from build123d import *

# Parameters (mm, degrees)
SKETCH7_R           = 15.75
BOSS_EXTRUDE5_DEPTH = 2
SKETCH8_R           = 0.8
BOSS_EXTRUDE6_DEPTH = 5


with BuildPart() as part:
    # Sketch7 → Boss-Extrude5 (new body)
    with BuildSketch(Plane(origin=(0, 0, 0), x_dir=(1, 0, 0), z_dir=(0, 1, 0))):
        with Locations(Location((0, 0, 0), (0, 0, 270))):
            Circle(SKETCH7_R)
    extrude(amount=BOSS_EXTRUDE5_DEPTH)

    # Sketch8 → Boss-Extrude6 (add)
    with BuildSketch(Plane.XZ):
        with Locations(Location((0, 14, 0), (0, 0, 90))):
            Circle(SKETCH8_R)
        with Locations(Location((14, 0, 0), (0, 0, 90))):
            Circle(SKETCH8_R)
        with Locations(Location((0, -14, 0), (0, 0, 90))):
            Circle(SKETCH8_R)
        with Locations(Location((-14, 0, 0), (0, 0, 90))):
            Circle(SKETCH8_R)
    extrude(amount=BOSS_EXTRUDE6_DEPTH)


solid = part.part
The listing builds one solid part. Answer for the finished solid, in the listing's coordinates (mm). A direction names the side the tool comes from. Round coordinates to 2 decimals unless told otherwise and drop trailing zeros. Write each loop counter-clockwise with the first axis right and the second up, starting at its lowest first coordinate (ties: lowest second). Pieces come first, ordered by that corner, then holes. Notation, with made-up numbers: (38.5, 56.5) - (77.5, 56.5) arc R13 cw to (77.5, 69.5) - close; hole circle Ø2 at (49, 19.5). An arc over 180 degrees is marked (long way). Use a Markdown table: item, result. Add a question column.
1. For a pull along Z with two mould halves and no side action, classify faces 3 (the face through (-14, -5, 0)), 4 (the face through (-0.54, -2.46, -14.59)), 5 (the face through (13.207, -2.465, -0.104)) as +Z half, -Z half, draft (parallel to the pull), parting line (faces both ways), or undercut.
2. The part is cut by section B-B (z = 0). Write down the section's boundary in (x, y), and give its area (3 significant figures).
3. A tool of negligible diameter and unlimited length cuts with its end or side. For faces 1 (the face through (15.616, 0.986, -2.05)), 2 (the face through (-0.54, -2.46, 13.41)), from which of +Z, -Z, +X, -X, +Y, -Y can it reach the whole face along a straight path? Write none if from no direction.
4. The part is cut by section C-C (y = -3.75). Write down the section's boundary in (x, z), and give its area (3 significant figures).
5. The part is cut by section D-D (y = 1). Write down the section's boundary in (x, z), and give its area (3 significant figures).
6. Consider line 1 (X direction, y = -2, z = 0); line 2 (Y direction, x = 10.5, z = 5); line 3 (X direction, y = -1, z = -14). Determine where each line is inside the solid, lowest interval first.
7. The part is cut by section A-A (x = 0). Write down the section's boundary in (y, z).
8. Flat-ended cylindrical pins translate along their axes: P1, Ø4, axis at x = -3, y = -0.5, coming from the +Z side; P2, Ø9.5, axis at x = 5, z = 7.5, coming from the -Y side; P3, Ø4, axis at x = 11.5, y = -2.5, coming from the -Z side. Find the tip coordinate at first contact, or state that the pin passes through.
Reported:
| question | item | result |
|---|---|---|
| 1 | face 3 | draft |
| 1 | face 4 | undercut |
| 1 | face 5 | parting line |
| 2 | outline | (-15.75, 0) - (-14.8, 0) - (-14.8, -5) - (-13.2, -5) - (-13.2, 0) - (13.2, 0) - (13.2, -5) - (14.8, -5) - (14.8, 0) - (15.75, 0) - (15.75, 2) - (-15.75, 2) - close |
| 2 | area | 79.0 mm^2 |
| 3 | face 1 | +Y, -Y |
| 3 | face 2 | -Y |
| 4 | outline | circle Ø1.6 at (-14, 0); circle Ø1.6 at (0, -14); circle Ø1.6 at (0, 14); circle Ø1.6 at (14, 0) |
| 4 | area | 8.04 mm^2 |
| 5 | outline | circle Ø31.5 at (0, 0) |
| 5 | area | 779 mm^2 |
| 6 | line 1 | -14.8 to -13.2, 13.2 to 14.8 |
| 6 | line 2 | 0 to 2 |
| 6 | line 3 | -0.8 to 0.8 |
| 7 | outline | (-5, -14.8) - (0, -14.8) - (0, -15.75) - (2, -15.75) - (2, 15.75) - (0, 15.75) - (0, 14.8) - (-5, 14.8) - (-5, 13.2) - (0, 13.2) - (0, -13.2) - (-5, -13.2) - close |
| 8 | P1 | z = 15.71 |
| 8 | P2 | y = 0 |
| 8 | P3 | z = -0.62 |
